Check sheet for the drawn part. Datum: minimum x, y, z corner. Units: mm. A direction names the side the tool comes from. Round coordinates to 2 decimals unless told otherwise and drop trailing zeros. Write each loop counter-clockwise with the first axis right and the second up, starting at its lowest first coordinate (ties: lowest second). Pieces come first, ordered by that corner, then holes.
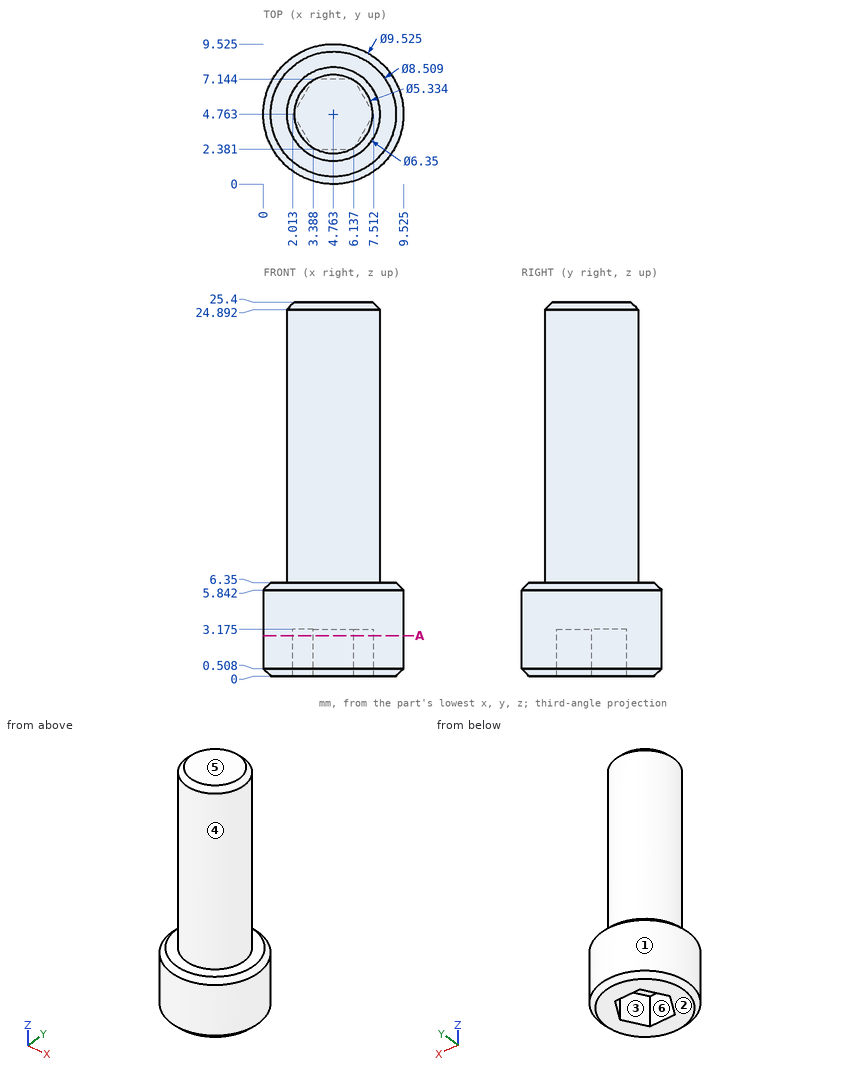
Q1. Depth check by flat-ended pin: P1, Ø4, axis at x = 4.5, z = 22, coming from the +Y side; P2, Ø1, axis at x = 2.5, z = 13, coming from the +Y side; P3, Ø3, axis at x = 8.5, z = 22.5, coming from the +Y side (1 decimal). Enter the tip coordinate at first touch or a pass-through.
Recorded:
P1: stops at y = 7.94
P2: stops at y = 7.4
P3: stops at y = 7
Q2. Material ranges on line 1 along Z through (x, y) = (8.25, 2.5); line 2 along Z through (x, y) = (4.75, 6) (1 decimal); line 3 along X through (y, z) = (5, 5.25) (1 decimal), recorded low to high.
Recorded:
line 1: z = 0 to 6.35
line 2: z = 3.2 to 25.4
line 3: x = 0 to 9.5
Q3. Release check for a two-part mould opening along X. For the marked faces 1, 2 and 3 record: released by +X, released by -X, zero draft, split by the parting line, or undercut.
Recorded:
face 1: split by the parting line
face 2: zero draft
face 3: undercut
Q4. Tool access check on the marked faces 4, 5 and 6. Record the directions out of +Z, -Z, +X, -X, +Y, -Y that give a thin tool (end or side, any length) a straight path to the whole face; none if there is none.
Recorded:
face 4: +Z
face 5: +Z, +X, -X, +Y, -Y
face 6: -Z
Q5. Sectioned sample at A-A (z = 2.75). Enter the section's corners in (x, y) (1 decimal).
Recorded:
outline: circle Ø9.5 at (4.8, 4.8); hole (2, 4.8) - (3.4, 2.4) - (6.1, 2.4) - (7.5, 4.8) - (6.1, 7.1) - (3.4, 7.1) - close
